Read the model definition and answer for the solid it produces. Units are mm, in the model's axes. A direction names the side the tool comes from. Give positions to 0.01 mm unless a question says otherwise; leave off trailing zeros. Order: outer loops, then holes, each group sorted by start corner. A loop starts at its lowest first (then second) coordinate and runs counter-clockwise, first axis right, second up.
```python
from build123d import *

# Parameters (mm, degrees)
SKETCH_1_W          = 10
SKETCH_1_H          = 8
EXTRUDE_1_DEPTH     = 6
EXTRUDE_2_DEPTH     = 45
CUT_EXTRUDE_1_REACH = 52.517
SKETCH_3_R          = 2.46


with BuildPart() as part:
    # 草图1 → 凸台-拉伸1 (new body)
    with BuildSketch(Plane(origin=(0, 0, 0), x_dir=(1, 0, 0), z_dir=(0, 1, 0))):
        Rectangle(SKETCH_1_W, SKETCH_1_H)
    extrude(amount=EXTRUDE_1_DEPTH)

    # 草图2 → 凸台-拉伸2 (add)
    with BuildSketch(Plane(origin=(5, 0, 0), x_dir=(0, 0, -1), z_dir=(1, 0, 0))):
        with BuildLine():
            ThreePointArc((0, 6), (-3, 3), (0, 0))
            Line((0, 0), (0, 6))
        make_face()
        with BuildLine():
            Line((0, 6), (0, 0))
            ThreePointArc((0, 0), (2.121320344, 0.878679656), (3, 3))
            ThreePointArc((3, 3), (2.121320344, 5.121320344), (0, 6))
        make_face()
    extrude(amount=EXTRUDE_2_DEPTH)

    # 草图3 → 切除-拉伸1 (cut, up to next)
    with BuildSketch(Plane(origin=(0, 6, 0), x_dir=(1, 0, 0), z_dir=(0, 1, 0)), mode=Mode.PRIVATE) as cut_extrude_1_sk1:
        with Locations(Location((-0.5, 0, 0), (0, 0, 270))):
            Circle(SKETCH_3_R)
    cut_extrude_1_tool1 = extrude(cut_extrude_1_sk1.sketch, amount=-CUT_EXTRUDE_1_REACH, mode=Mode.PRIVATE) & part.part
    add(cut_extrude_1_tool1.solids().sort_by_distance((-0.5, 6, 0))[0], mode=Mode.SUBTRACT)


solid = part.part
```
1) The part is cut by section D-D on x = 13. Determine the outline of the cut face in (y, z), and give its area (3 significant figures).
Final values:
outline: circle Ø6 at (3, 0)
area: 28.3 mm2
2) The part is cut by section C-C on z = 1.25. Determine the outline of the cut face in (x, y).
Final values:
outline: (-5, 0) - (-2.62, 0) - (-2.62, 6) - (-5, 6) - close; (1.62, 0) - (5, 0) - (5, 0.27) - (50, 0.27) - (50, 5.73) - (5, 5.73) - (5, 6) - (1.62, 6) - close
3) A tool of negligible diameter and unlimited length cuts with its end or side. For faces 1 (the face through (5, 3, 3.4)), 2 (the face through (2.2, 6, -0.1)), 3 (the face through (5, 3, -3.3)), from which of +Z, -Z, +X, -X, +Y, -Y can it reach the whole face along a straight path? Write none if from no direction.
Final values:
face 1: +Z, +X
face 2: +Z, -Z, +X, -X, +Y
face 3: -Z, +X
4) The part is cut by section A-A on y = 4.8. Determine the outline of the cut face in (x, z), and give its area (3 significant figures).
Final values:
outline: (-5, -4) - (5, -4) - (5, -2.4) - (50, -2.4) - (50, 2.4) - (5, 2.4) - (5, 4) - (-5, 4) - close; hole circle Ø4.92 at (-0.5, 0)
area: 277 mm2
5) For a pull along Z with two mould halves and no side action, classify faces 4 (the face through (0, 3, -4)), 5 (the face through (0, 3, 4)), 6 (the face through (1.574, 3.042, 1.322)) as released by +Z, released by -Z, zero draft, split by the parting line, or undercut.
Final values:
face 4: released by -Z
face 5: released by +Z
face 6: undercut
6) The part is cut by section B-B on x = -0.5. Determine the outline of the cut face in (y, z).
Final values:
outline: (0, -4) - (6, -4) - (6, -2.46) - (0, -2.46) - close; (0, 2.46) - (6, 2.46) - (6, 4) - (0, 4) - close
7) Consider L1, parallel to X at y = 5.5, z = 0; L2, parallel to X at y = 1.4, z = 3.5; L3, parallel to X at y = 0.6, z = 1.5. Determine where each line is inside the solid, lowest interval first.
Final values:
L1: x = -5 to -2.96, 1.96 to 50
L2: x = -5 to 5
L3: x = -5 to -2.45, 1.45 to 50
